```python
from build123d import *

# Parameters (mm, degrees)
PAD_DEPTH = 1


with BuildPart() as obj1:
    # Sketch → Revolution (revolve)
    with BuildSketch(Plane.XZ):
        Polygon((0, 0), (0, 1.511325), (-0.5, 1.8), (-1.67, 1.8), (-1.77, 1.7), (-1.77, 0.85), (-2.92, 0.85), (-2.92, 1.7), (-3.02, 1.8), (-4.2, 1.8), (-4.7, 1.511325), (-4.7, 0), align=None)
    revolve(axis=Axis((0, 0, 0), (1, 0, 0)))


with BuildPart() as body004:
    # Body004 base: copy of obj1
    add(obj1.part)


with BuildPart() as body004_1:
    # Body004 placement: moved
    add(body004.part.moved(Location((0, 0, 40))))


with BuildPart() as body010:
    # Body010 base: copy of Body004
    add(body004_1.part)


with BuildPart() as body010_1:
    # Body010 placement: moved
    add(body010.part.moved(Location((0, 10, 0))))


with BuildPart() as body003:
    # Body003 base: copy of obj1
    add(obj1.part)


with BuildPart() as body003_1:
    # Body003 placement: moved
    add(body003.part.moved(Location((0, 0, 30))))


with BuildPart() as body009:
    # Body009 base: copy of Body003
    add(body003_1.part)


with BuildPart() as body009_1:
    # Body009 placement: moved
    add(body009.part.moved(Location((0, 10, 0))))


with BuildPart() as body002:
    # Body002 base: copy of obj1
    add(obj1.part)


with BuildPart() as body002_1:
    # Body002 placement: moved
    add(body002.part.moved(Location((0, 0, 20))))


with BuildPart() as body008:
    # Body008 base: copy of Body002
    add(body002_1.part)


with BuildPart() as body008_1:
    # Body008 placement: moved
    add(body008.part.moved(Location((0, 10, 0))))


with BuildPart() as body006:
    # Body006 base: copy of obj1
    add(obj1.part)


with BuildPart() as body006_1:
    # Body006 placement: moved
    add(body006.part.moved(Location((0, 10, 0))))


with BuildPart() as body001:
    # Body001 base: copy of obj1
    add(obj1.part)


with BuildPart() as body001_1:
    # Body001 placement: moved
    add(body001.part.moved(Location((0, 0, 10))))


with BuildPart() as body007:
    # Body007 base: copy of Body001
    add(body001_1.part)


with BuildPart() as body007_1:
    # Body007 placement: moved
    add(body007.part.moved(Location((0, 10, 0))))


with BuildPart() as obj2:
    # Sketch002 → Pad (new body)
    with BuildSketch(Plane.YZ.offset(-0.6)):
        Polygon((0, -0.25), (10.25, -0.25), (10.25, 10.25), (0.25, 10.25), (0.25, 19.75), (10.25, 19.75), (10.25, 30.25), (0.25, 30.25), (0.25, 39.75), (10, 39.75), (10, 40.25), (-0.25, 40.25), (-0.25, 29.75), (9.75, 29.75), (9.75, 20.25), (-0.25, 20.25), (-0.25, 9.75), (9.75, 9.75), (9.75, 0.25), (0, 0.25), (0, 0), align=None)
    extrude(amount=-PAD_DEPTH)

    # Boolean: union Body010, Body009, Body008, Body006, Body007, Body004, Body002, Body003, Body001, obj1
    add(body010_1.part)
    add(body009_1.part)
    add(body008_1.part)
    add(body006_1.part)
    add(body007_1.part)
    add(body004_1.part)
    add(body002_1.part)
    add(body003_1.part)
    add(body001_1.part)
    add(obj1.part)


solid = obj2.part
```
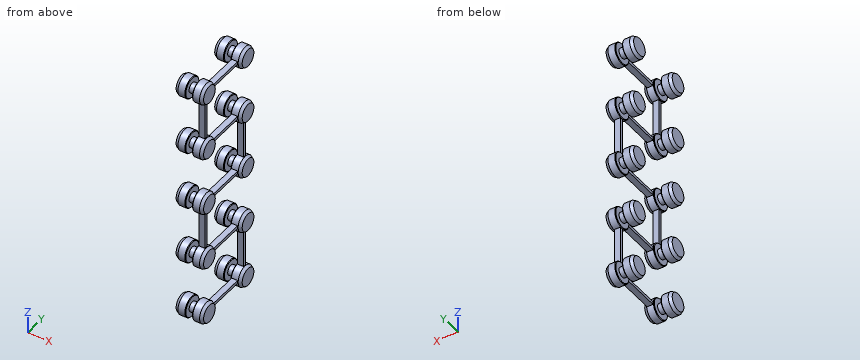
Work out the finished part from the listing and answer in its coordinate system (mm). Round coordinates to 2 decimals unless told otherwise and drop trailing zeros. Order: outer loops, then holes, each group sorted by start corner. A loop starts at its lowest first (then second) coordinate and runs counter-clockwise, first axis right, second up.
Q1. A cutting plane is placed at A-A, the plane y = 3.25. Determine the outline of the cut face in (x, z), then the cut area to 3 significant figures.
Solution:
outline: (-1.6, -0.25) - (-0.6, -0.25) - (-0.6, 0.25) - (-1.6, 0.25) - close; (-1.6, 9.75) - (-0.6, 9.75) - (-0.6, 10.25) - (-1.6, 10.25) - close; (-1.6, 19.75) - (-0.6, 19.75) - (-0.6, 20.25) - (-1.6, 20.25) - close; (-1.6, 29.75) - (-0.6, 29.75) - (-0.6, 30.25) - (-1.6, 30.25) - close; (-1.6, 39.75) - (-0.6, 39.75) - (-0.6, 40.25) - (-1.6, 40.25) - close
area: 2.50 mm2
Q2. Find the intervals of material crossed by line 1 along Z through (x, y) = (-3.7, 1.25); line 2 along X through (y, z) = (-0.75, 39); line 3 along Z through (x, y) = (-3.75, 0.75), in increasing order.
Solution:
line 1: z = -1.3 to 1.3, 8.7 to 11.3, 18.7 to 21.3, 28.7 to 31.3, 38.7 to 41.3
line 2: x = -4.7 to -2.92, -1.77 to 0
line 3: z = -1.64 to 1.64, 8.36 to 11.64, 18.36 to 21.64, 28.36 to 31.64, 38.36 to 41.64
Q3. A cutting plane is placed at B-B, the plane z = 5.5. Determine the outline of the cut face in (x, y), then the cut area to 3 significant figures.
Solution:
outline: (-1.6, 9.75) - (-0.6, 9.75) - (-0.6, 10.25) - (-1.6, 10.25) - close
area: 0.500 mm2
Q4. Given pin 1 Ø4 at (y, z) = (6.5, 3) entering from +X; pin 2 Ø1.1 at (x, z) = (-1, 4) entering from -Y; pin 3 Ø0.6 at (y, z) = (10, 23.5) entering from +X; pin 4 Ø0.5 at (x, z) = (-1, 14.5) entering from +Y, each flat-ended and moving along its own axis, determine where each tip first touches the part or whether it passes through.
Solution:
pin 1: passes through
pin 2: stops at y = 9.75
pin 3: stops at x = -0.6
pin 4: stops at y = 0.25
